```python
from build123d import *

# Parameters (mm, degrees)
EXTRUDE_1_DEPTH = 10


with BuildPart() as part:
    # 草图1 → 凸台-拉伸1 (new body)
    with BuildSketch(Plane.XY):
        Polygon((-65, 0), (-45, -20), (-45, -71.366959064), (65, -71.366959064), (65, 71.366959064), (-65, 71.366959064), align=None)
        Polygon((45, 56.366959064), (-45, 56.366959064), (-45, 16.366959064), (-35, 6.366959064), (45, 6.366959064), align=None, mode=Mode.SUBTRACT)
        with BuildLine():
            Line((20, -21.366959064), (-20, -21.366959064))
            ThreePointArc((-20, -21.366959064), (-27.071067812, -24.295891252), (-30, -31.366959064))
            Line((-30, -31.366959064), (-30, -41.366959064))
            ThreePointArc((-30, -41.366959064), (-27.071067812, -48.438026876), (-20, -51.366959064))
            Line((-20, -51.366959064), (20, -51.366959064))
            ThreePointArc((20, -51.366959064), (27.071067812, -48.438026876), (30, -41.366959064))
            Line((30, -41.366959064), (30, -31.366959064))
            ThreePointArc((30, -31.366959064), (27.071067812, -24.295891252), (20, -21.366959064))
        make_face(mode=Mode.SUBTRACT)
    extrude(amount=EXTRUDE_1_DEPTH)


solid = part.part
```
Geometry check sheet. Reference: the model listing, model coordinates, mm. A direction names the side the tool comes from. Give positions to 0.01 mm unless a question says otherwise; leave off trailing zeros. Write each loop counter-clockwise with the first axis right and the second up, starting at its lowest first coordinate (ties: lowest second). Pieces come first, ordered by that corner, then holes. Notation, with made-up numbers: (-10, -17) -> (19, -17) arc R15 cw to (19, -4) -> close; hole circle Ø4 at (29.5, 42.5). An arc over 180 degrees is marked (long way). One line per question, with ' | ' between items.
Item 1: Depth check by flat-ended pin: pin 1 (4 mm diameter, centred on y = -40, z = 8.5, fed in from -X); pin 2 (3 mm diameter, centred on x = 28, y = -25.5, fed in from +Z). Enter the tip coordinate at first touch or a pass-through.
Determined:
pin 1: x = -45 | pin 2: z = 10
Item 2: Sectioned sample at B-B, the plane x = -43. Record the boundary of the cut face in (y, z), plus the area to 3 significant figures.
Determined:
outline: (-71.37, 0) -> (14.37, 0) -> (14.37, 10) -> (-71.37, 10) -> close; (56.37, 0) -> (71.37, 0) -> (71.37, 10) -> (56.37, 10) -> close | area: 1,010 mm^2
Item 3: Sectioned sample at A-A, the plane y = 21. Record the boundary of the cut face in (x, z).
Determined:
outline: (-65, 0) -> (-45, 0) -> (-45, 10) -> (-65, 10) -> close; (45, 0) -> (65, 0) -> (65, 10) -> (45, 10) -> close
Item 4: Draft check along Z on faces 3 (the flat face through (-1, 1, 0)), 4 (the flat face through (0, -51.367, 5)). Enter one of: released by +Z, released by -Z, zero draft, split by the parting line, or undercut.
Determined:
face 3: released by -Z | face 4: zero draft
Item 5: Sectioned sample at C-C, the plane z = 4.5. Record the boundary of the cut face in (x, y), plus the area to 3 significant figures.
Determined:
outline: (-65, 0) -> (-45, -20) -> (-45, -71.37) -> (65, -71.37) -> (65, 71.37) -> (-65, 71.37) -> close; hole (-45, 16.37) -> (-35, 6.37) -> (45, 6.37) -> (45, 56.37) -> (-45, 56.37) -> close; hole (-30, -41.37) arc R10 ccw to (-20, -51.37) -> (20, -51.37) arc R10 ccw to (30, -41.37) -> (30, -31.37) arc R10 ccw to (20, -21.37) -> (-20, -21.37) arc R10 ccw to (-30, -31.37) -> close | area: 11,200 mm^2
Item 6: Access from +Z, -Z, +X, -X, +Y, -Y to the whole of each face (thin tool, end or side, straight path). Record for faces 1 (the flat face through (30, -36, 5)), 2 (the flat face through (-55, -10, 5)).
Determined:
face 1: +Z, -Z | face 2: +Z, -Z, -X, -Y
Item 7: Scan lines: line 1 along Y through (x, z) = (2.5, 9.5); line 2 along X through (y, z) = (43, 0.75); line 3 along Y through (x, z) = (41, 5.5). Record each from-to range of solid material in increasing order.
Determined:
line 1: -71.37 to -51.37, -21.37 to 6.37, 56.37 to 71.37 | line 2: -65 to -45, 45 to 65 | line 3: -71.37 to 6.37, 56.37 to 71.37
Item 8: Sectioned sample at D-D, the plane x = -24. Record the boundary of the cut face in (y, z), plus the area to 3 significant figures.
Determined:
outline: (-71.37, 0) -> (-50.53, 0) -> (-50.53, 10) -> (-71.37, 10) -> close; (-22.2, 0) -> (6.37, 0) -> (6.37, 10) -> (-22.2, 10) -> close; (56.37, 0) -> (71.37, 0) -> (71.37, 10) -> (56.37, 10) -> close | area: 644 mm^2
